```python
from build123d import *

# Parameters (mm, degrees)
CHAMFER1_SIZE         = 1
SKETCH2_R             = 6
BOSS_EXTRUDE1_DEPTH   = 15
CHAMFER2_SIZE         = 0.5
F_5_0MM_DOWEL_HOLE1_D = 5


with BuildPart() as part:
    # Sketch1 → Revolve1 (revolve)
    with BuildSketch(Plane.XY, mode=Mode.PRIVATE) as revolve1_sk:
        Polygon((2.5, 15.517957554), (6, 15.517957554), (8.853571596, -0.66545116), (12, -2.482042446), (12, -4.482042446), (11.116055663, -4.482042446), (10.718293105, -3.566194226), (9.374682102, -4.487525743), (7.83057192, -3.153662628), (6.678328492, -4.487525743), (4.849032939, -4.487525743), (3.335400026, -4.487525743), (2.39653501, -3.879149231), (1.705781249, -4.482042446), (0, -4.482042446), (0, 0), (2.5, 0), align=None)
    revolve(revolve1_sk.sketch.rotate(Axis((0, -4.482042446, 0), (0, 1, 0)), 90), axis=Axis((0, -4.482042446, 0), (0, 1, 0)))

    # Chamfer1
    chamfer1_edges = [part.edges().sort_by_distance(p)[0] for p in [
        (0, 15.517957554, 2.5),
    ]]
    chamfer(chamfer1_edges, length=CHAMFER1_SIZE)

    # Sketch2 → Boss-Extrude1 (add)
    with BuildSketch(Plane(origin=(0, 15.517957554, 0), x_dir=(1, 0, 0), z_dir=(0, 1, 0))):
        Polygon((0, 8.082903769), (-7, 4.041451884), (-7, -4.041451884), (0, -8.082903769), (7, -4.041451884), (7, 4.041451884), align=None)
        Circle(SKETCH2_R, mode=Mode.SUBTRACT)
    extrude(amount=-BOSS_EXTRUDE1_DEPTH)

    # Chamfer2
    chamfer2_edges = [part.edges().sort_by_distance(p)[0] for p in [
        (3.5, 15.517957554, -6.062177826),
        (-3.5, 15.517957554, -6.062177826),
        (-7, 15.517957554, 0),
        (-3.5, 15.517957554, 6.062177826),
        (3.5, 15.517957554, 6.062177826),
        (7, 15.517957554, 0),
    ]]
    chamfer(chamfer2_edges, length=CHAMFER2_SIZE)

    # Ø5.0mm Dowel Hole1 (through all)
    with Locations(Plane(origin=(0, -4.482042446, 0), x_dir=(-1, 0, 0), z_dir=(0, -1, 0))):
        with Locations((0, 0)):
            Hole(F_5_0MM_DOWEL_HOLE1_D / 2)


solid = part.part
```
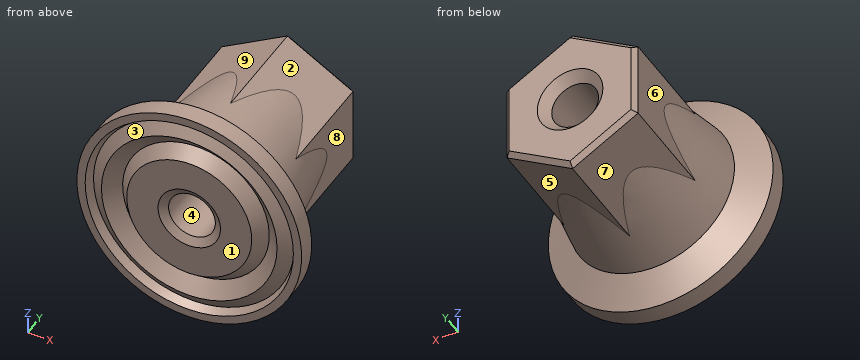
Part model, mm, in its own coordinate system. Face numbers are marked on the shaded views. A direction names the side the tool comes from. Give positions to 0.01 mm unless a question says otherwise; leave off trailing zeros. Order: outer loops, then holes, each group sorted by start corner. A loop starts at its lowest first (then second) coordinate and runs counter-clockwise, first axis right, second up. Notation, with made-up numbers: M 27.25,55.5 L 77.25,55.5 A26 cw 77.25,90.5 Z; hole C 65.5,11 d10. An arc over 180 degrees is marked long. Use a Markdown table: item, result. Add a question column.
(1) Saw through at A-A, the plane y = 6.25. Give the cut face in (x, z).
(2) Drop flat-ended pins along their axis: P1, Ø12, axis at x = 6.5, y = -0.5, coming from the -Z side; P2, Ø6.5, axis at y = 11, z = -0.5, coming from the +X side; P3, Ø3, axis at x = 9, z = 9.5, coming from the -Y side. Give the stop position or say it passes through.
(3) Saw through at B-B, the plane y = 2.5. Give the cut face in (x, z), and give its area (3 significant figures).
(4) Probe line 1 along Z through (x, y) = (-3.25, -3.25); line 2 along X through (y, z) = (14.25, 0); line 3 along X through (y, z) = (3.5, 0). List the from-to ranges inside material, lowest first. Write a range as [from, to].
(5) Mould opens along X. For the marked faces 1, 2, 3 and 4 say: +X half, -X half, draft (parallel to the pull), parting line (faces both ways), or undercut.
(6) 3-axis set-ups, long thin cutter, end or side, ignore diameter. For the marked faces 5, 6, 7, 8 and 9: which of +Z, -Z, +X, -X, +Y, -Y reach the whole face in a straight line?
Answer key:
| question | item | result |
|---|---|---|
| 1 | outline | M -7,-4.04 L -6.14,-4.54 A7.63 ccw -0.86,-7.59 L 0,-8.08 L 0.86,-7.59 A7.63 ccw 6.14,-4.54 L 7,-4.04 L 7,-3.05 A7.63 ccw 7,3.05 L 7,4.04 L 6.14,4.54 A7.63 ccw 0.86,7.59 L 0,8.08 L -0.86,7.59 A7.63 ccw -6.14,4.54 L -7,4.04 L -7,3.05 A7.63 ccw -7,-3.05 Z; hole C 0,0 d5 |
| 2 | P1 | z = -11.97 |
| 2 | P2 | x = 7.36 |
| 2 | P3 | y = -4.48 |
| 3 | outline | C 0,0 d16.59; hole C 0,0 d5 |
| 3 | area | 197 mm^2 |
| 4 | line 1 | [-11.55, -7.25], [-7.03, 7.03], [7.25, 11.55] |
| 4 | line 2 | [-7, -2.5], [2.5, 7] |
| 4 | line 3 | [-8.12, -2.5], [2.5, 8.12] |
| 5 | face 1 | draft |
| 5 | face 2 | +X half |
| 5 | face 3 | undercut |
| 5 | face 4 | undercut |
| 6 | face 5 | -Z, +X, +Y |
| 6 | face 6 | -X, +Y |
| 6 | face 7 | -Z, -X, +Y |
| 6 | face 8 | +X, +Y |
| 6 | face 9 | +Z, -X, +Y |
